from build123d import *

# Parameters (mm, degrees)
SKETCH1_R           = 3.1115
BOSS_EXTRUDE1_DEPTH = 19.05
SKETCH2_R           = 8.255
SKETCH2_R_2         = 3.1115
BOSS_EXTRUDE2_DEPTH = 19.05
FILLET1_R           = 2.54


with BuildPart() as part:
    # Sketch1 → Boss-Extrude1 (new body)
    with BuildSketch(Plane(origin=(0, 0, 0), x_dir=(1, 0, 0), z_dir=(0, 1, 0))):
        with BuildLine():
            Line((-80.645, -8.255), (80.645, -8.255))
            ThreePointArc((80.645, -8.255), (88.9, 0), (80.645, 8.255))
            Line((80.645, 8.255), (-80.645, 8.255))
            ThreePointArc((-80.645, 8.255), (-88.9, 0), (-80.645, -8.255))
        make_face()
        with Locations((-80.645, 0)):
            Circle(SKETCH1_R, mode=Mode.SUBTRACT)
        with Locations((80.645, 0)):
            Circle(SKETCH1_R, mode=Mode.SUBTRACT)
    extrude(amount=BOSS_EXTRUDE1_DEPTH)

    # Sketch2 → Boss-Extrude2 (add)
    with BuildSketch(Plane(origin=(0, 19.05, 0), x_dir=(1, 0, 0), z_dir=(0, 1, 0))):
        with Locations((-23.650230322, -9.8425)):
            Circle(SKETCH2_R)
        with Locations((-23.650230322, -11.43)):
            Circle(SKETCH2_R_2, mode=Mode.SUBTRACT)
    extrude(amount=-BOSS_EXTRUDE2_DEPTH)

    # Fillet1
    fillet1_edges = [part.edges().sort_by_distance(p)[0] for p in [
        (88.9, 19.05, 0),
        (0, 19.05, -8.255),
        (32.547843725, 0, 8.255),
        (32.547843725, 19.05, 8.255),
        (-23.650230322, 19.05, 18.0975),
        (-23.650230322, 0, 18.0975),
        (-88.9, 19.05, 0),
        (0, 0, -8.255),
        (88.9, 0, 0),
        (-56.198074047, 0, 8.255),
        (-88.9, 0, 0),
        (-56.198074047, 19.05, 8.255),
    ]]
    fillet(fillet1_edges, radius=FILLET1_R)


solid = part.part
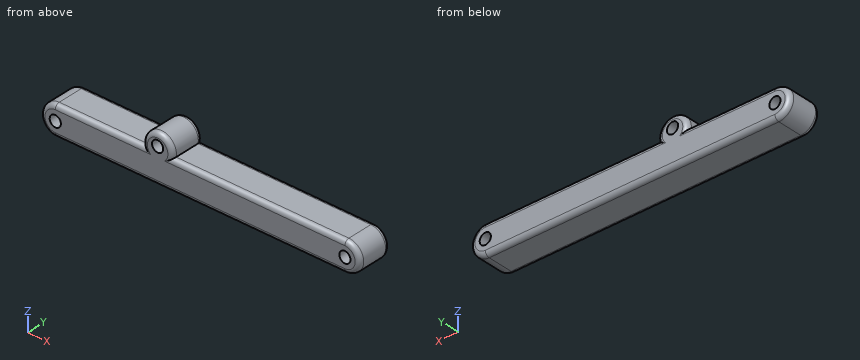
Could you check a few things on this model? Use its own coordinates, in mm. Coordinates: 2 decimals unless noted, no trailing zeros. Write each loop counter-clockwise with the first axis right and the second up, starting at its lowest first coordinate (ties: lowest second). Pieces come first, ordered by that corner, then holes. Notation, with made-up numbers: M 88,67.25 L 141,67.25 A23 cw 141,104.25 Z; hole C 73.25,-28.5 d11. An arc over 180 degrees is marked long. One line per question, with ' | ' between items.
1) Imagine slicing it at B-B, the plane z = 0. Write out the boundary of the cut face in (x, y).
Checks:
outline: M -88.9,2.54 A2.54 ccw -86.36,0 L -83.76,0 L -83.76,19.05 L -86.36,19.05 A2.54 ccw -88.9,16.51 Z; M -77.53,0 L 77.53,0 L 77.53,19.05 L -77.53,19.05 Z; M 83.76,0 L 86.36,0 A2.54 ccw 88.9,2.54 L 88.9,16.51 A2.54 ccw 86.36,19.05 L 83.76,19.05 Z
2) Imagine slicing it at C-C, the plane x = -66.5. Write out the boundary of the cut face in (y, z) (3 decimals).
Checks:
outline: M 0,-5.715 A2.54 ccw 2.54,-8.255 L 16.51,-8.255 A2.54 ccw 19.05,-5.715 L 19.05,5.715 A2.54 ccw 16.51,8.255 L 2.54,8.255 A2.54 ccw 0,5.715 Z
3) Imagine slicing it at A-A, the plane y = 4.75. Write out the boundary of the cut face in (x, z) (1 decimal).
Checks:
outline: M -80.6,-8.3 L 80.6,-8.3 A8.3 ccw 80.6,8.3 L -15.5,8.3 A8.3 ccw long -31.8,8.3 L -80.6,8.3 A8.3 ccw Z; hole C -80.6,0 d6.2; hole C -23.7,11.4 d6.2; hole C 80.6,0 d6.2
4) I need wall thicknesses on probe 1 along X at (y, z) = (14.5, 0); probe 2 along X at (y, z) = (15, 11.43); probe 3 along Z at (x, y) = (9, 3.5) (3 decimals). Which ranges of each line are inside material? Lowest first, please. Write a range as [from, to].
Checks:
probe 1: [-88.9, -83.76], [-77.53, 77.53], [83.76, 88.9] | probe 2: [-31.75, -26.76], [-20.54, -15.55] | probe 3: [-8.255, 8.255]
5) For pin 1 Ø7 at (x, z) = (-80.645, 0) entering from -Y; pin 2 Ø10 at (y, z) = (8, 9) entering from +X; pin 3 Ø7 at (x, y) = (48.5, 11.5) entering from +Z (3 decimals), each with a flat end and sliding along its axis, tell me the tip position at first contact or that it passes through.
Checks:
pin 1: y = 0 | pin 2: x = 87.87 | pin 3: z = 8.255
